```python
from build123d import *

# Parameters (mm, degrees)
SKETCH1_R           = 1.5
BOSS_EXTRUDE1_DEPTH = 4


with BuildPart() as part:
    # Sketch1 → Boss-Extrude1 (new body)
    with BuildSketch(Plane.XY):
        with BuildLine():
            Line((15.238123377, 6.19825268), (16.347575878, 4.533215952))
            ThreePointArc((16.347575878, 4.533215952), (16.410300459, 4.443659946), (16.477115989, 4.357113217))
            ThreePointArc((16.477115989, 4.357113217), (16.486629929, 4.345440812), (16.496218344, 4.333829508))
            ThreePointArc((16.496218344, 4.333829508), (19.970988274, 4.173992248), (19.811151014, 7.648762179))
            ThreePointArc((19.811151014, 7.648762179), (19.79953971, 7.658350594), (19.787867306, 7.667864534))
            ThreePointArc((19.787867306, 7.667864534), (19.701320577, 7.734680065), (19.61176457, 7.797404645))
            Line((19.61176457, 7.797404645), (17.946727843, 8.906857145))
            ThreePointArc((17.946727843, 8.906857145), (17.307596881, 9.783053451), (17.389325425, 10.864501))
            ThreePointArc((17.389325425, 10.864501), (17.507217214, 11.135394708), (17.61540591, 11.410307569))
            ThreePointArc((17.61540591, 11.410307569), (18.322313997, 12.232797271), (19.393812184, 12.400427786))
            Line((19.393812184, 12.400427786), (21.601765932, 11.971688999))
            ThreePointArc((21.601765932, 11.971688999), (24.171821324, 14.31570037), (21.601765932, 16.65971174))
            Line((21.601765932, 16.65971174), (19.393812182, 16.230972956))
            ThreePointArc((19.393812182, 16.230972956), (18.322313995, 16.398603469), (17.615405908, 17.221093173))
            ThreePointArc((17.615405908, 17.221093173), (17.507217213, 17.496006033), (17.389325429, 17.766899742))
            ThreePointArc((17.389325429, 17.766899742), (17.307596884, 18.848347289), (17.946727842, 19.724543597))
            Line((17.946727842, 19.724543597), (19.61176457, 20.833996096))
            ThreePointArc((19.61176457, 20.833996096), (19.701320577, 20.896720677), (19.787867306, 20.963536208))
            ThreePointArc((19.787867306, 20.963536208), (19.79953971, 20.973050148), (19.811151014, 20.982638563))
            ThreePointArc((19.811151014, 20.982638563), (19.970988274, 24.457408494), (16.496218344, 24.297571234))
            ThreePointArc((16.496218344, 24.297571234), (16.486629929, 24.28595993), (16.477115989, 24.274287526))
            ThreePointArc((16.477115989, 24.274287526), (16.410300458, 24.187740797), (16.347575878, 24.09818479))
            Line((16.347575878, 24.09818479), (15.238123378, 22.433148063))
            ThreePointArc((15.238123378, 22.433148063), (14.36192707, 21.794017099), (13.280479519, 21.875745645))
            ThreePointArc((13.280479519, 21.875745645), (13.108222359, 21.952034546), (12.93428015, 22.024399135))
            Line((12.93428015, 22.024399135), (12.93428015, 43.31570037))
            ThreePointArc((12.93428015, 43.31570037), (9.82928015, 46.42070037), (6.72428015, 43.31570037))
            Line((6.72428015, 43.31570037), (6.72428015, 23.645064295))
            ThreePointArc((6.72428015, 23.645064295), (0.015567267, 13.708167902), (7.898674921, 4.674599826))
            Line((7.898674921, 4.674599826), (7.521150189, 2.789308191))
            ThreePointArc((7.521150189, 2.789308191), (7.502177507, 2.681629554), (7.488225443, 2.57318606))
            ThreePointArc((7.488225443, 2.57318606), (7.486699178, 2.558205052), (7.485268779, 2.543214587))
            ThreePointArc((7.485268779, 2.543214587), (9.82928015, -0.026840804), (12.173291521, 2.543214587))
            ThreePointArc((12.173291521, 2.543214587), (12.171861122, 2.558205052), (12.170334857, 2.57318606))
            ThreePointArc((12.170334857, 2.57318606), (12.156382793, 2.681629555), (12.137410113, 2.789308193))
            Line((12.137410113, 2.789308193), (11.744552736, 4.751168341))
            ThreePointArc((11.744552736, 4.751168341), (11.912183252, 5.822666526), (12.734672953, 6.529574612))
            ThreePointArc((12.734672953, 6.529574612), (13.009585814, 6.637763307), (13.280479523, 6.755655094))
            ThreePointArc((13.280479523, 6.755655094), (14.361927069, 6.837383639), (15.238123377, 6.19825268))
        make_face()
        with Locations((9.82928015, 14.31570037)):
            Circle(SKETCH1_R, mode=Mode.SUBTRACT)
        with Locations((9.82928015, 43.31570037)):
            Circle(SKETCH1_R, mode=Mode.SUBTRACT)
    extrude(amount=BOSS_EXTRUDE1_DEPTH)


solid = part.part
```
Model file for the job. Use its own axes, mm. A direction names the side the tool comes from. Coordinates: 2 decimals unless noted, no trailing zeros. Order: outer loops, then holes, each group sorted by start corner. A loop starts at its lowest first (then second) coordinate and runs counter-clockwise, first axis right, second up. Notation, with made-up numbers: (68, -17.75) - (92, -17.75) arc R37 cw to (92, 21.25) - close; hole circle Ø9 at (-10, -6.5). An arc over 180 degrees is marked (long way). Return JSON: item names as keys, results as strings. Group by question number.
1) Tool access for faces 4 (the flat face through (15.8, 23.28, 1.97)), 5 (the flat face through (20.48, 12.19, 1.97)), 6 (the flat face through (18.791, 8.344, 1.972)): list every direction of +Z, -Z, +X, -X, +Y, -Y with a clear straight run to the whole face (end or side of a thin tool).
2) Mould opens along Y. For faces 1 (the flat face through (7.713, 3.745, 1.972)), 2 (the flat face through (12, 18, 0)), 3 (the cylindrical face through (14.35, 6.84, 1.97)) say: released by +Y, released by -Y, zero draft, split by the parting line, or undercut.
3) Probe line 1 (Y direction, x = 10, z = 1.4); line 2 (Y direction, x = 19, z = 3.7); line 3 (X direction, y = 30, z = 0.7). List the from-to ranges inside material, lowest first. Write a range as from..to.
4) Saw through at C-C, the plane z = 0.9. Count the separate pieces of the cut face and the enclosed holes in it, plus the area to 3 significant figures.
5) Saw through at A-A, the plane y = 31.5. Write the cut outline in (x, z), plus the area to 3 significant figures.
6) Saw through at B-B, the plane x = 5. Write the cut outline in (y, z).
7) Flat gauge pins, fed straight in: P1, Ø10, axis at x = 20.5, y = 6.5, coming from the -Z side; P2, Ø1.2, axis at y = 28.5, z = 2, coming from the -X side. Where does each tip first touch, or does it go through?
Values found:
{
 "1": {"face 4": "+Z, -Z, +Y", "face 5": "+Z, -Z", "face 6": "+Z, -Z, +X"},
 "2": {"face 1": "undercut", "face 2": "zero draft", "face 3": "released by -Y"},
 "3": {"line 1": "y = -0.02..12.83, 15.81..41.83, 44.81..46.42", "line 2": "y = 3.59..8.21, 12.43..16.2, 20.43..25.04", "line 3": "x = 6.72..12.93"},
 "4": {"separate pieces": "1", "enclosed holes": "2", "area": "482 mm²"},
 "5": {"outline": "(6.72, 0) - (12.93, 0) - (12.93, 4) - (6.72, 4) - close", "area": "24.8 mm²"},
 "6": {"outline": "(5.75, 0) - (22.88, 0) - (22.88, 4) - (5.75, 4) - close"},
 "7": {"P1": "stops at z = 0", "P2": "stops at x = 6.72"}
}
